from build123d import *

# Parameters (mm, degrees)
SKETCH1_W           = 58
SKETCH1_H           = 90
SKETCH1_W_2         = 46
SKETCH1_H_2         = 78
BOSS_EXTRUDE1_DEPTH = 3
BOSS_EXTRUDE2_DEPTH = 6
SKETCH3_R           = 2.05
CUT_EXTRUDE1_DEPTH  = 108.447661678
SKETCH4_R           = 2.05
CUT_EXTRUDE2_DEPTH  = 108.447661678
FILLET1_R           = 2
FILLET2_R           = 2
SKETCH5_W           = 8
SKETCH5_H           = 3
BOSS_EXTRUDE3_DEPTH = 3
SKETCH6_R           = 2.05
CUT_EXTRUDE3_DEPTH  = 3
FILLET3_R           = 3
SKETCH7_W           = 3
SKETCH7_H           = 8
BOSS_EXTRUDE4_DEPTH = 3
SKETCH8_R           = 2.05
CUT_EXTRUDE4_DEPTH  = 108.238052948
FILLET4_R           = 3


with BuildPart() as part:
    # Sketch1 → Boss-Extrude1 (new body)
    with BuildSketch(Plane(origin=(0, 0, 0), x_dir=(1, 0, 0), z_dir=(0, 1, 0))):
        with Locations((29, -45)):
            Rectangle(SKETCH1_W, SKETCH1_H)
        with Locations((29, -45)):
            Rectangle(SKETCH1_W_2, SKETCH1_H_2, mode=Mode.SUBTRACT)
    extrude(amount=BOSS_EXTRUDE1_DEPTH)

    # Sketch2 → Boss-Extrude2 (add)
    with BuildSketch(Plane(origin=(0, 3, 0), x_dir=(1, 0, 0), z_dir=(0, 1, 0))):
        Polygon((46, -84), (46, -90), (58, -90), (58, -78), (52, -78), (52, -84), align=None)
        Polygon((52, -12), (58, -12), (58, 0), (46, 0), (46, -6), (52, -6), align=None)
        Polygon((0, 0), (0, -12), (6, -12), (6, -6), (12, -6), (12, 0), align=None)
        Polygon((0, -90), (12, -90), (12, -84), (6, -84), (6, -78), (0, -78), align=None)
    extrude(amount=BOSS_EXTRUDE2_DEPTH)

    # Sketch3 → Cut-Extrude1 (cut, through all)
    with BuildSketch(Plane.ZY):
        with Locations((9, 6)):
            Circle(SKETCH3_R)
        with Locations((81, 6)):
            Circle(SKETCH3_R)
    extrude(amount=-CUT_EXTRUDE1_DEPTH, mode=Mode.SUBTRACT)

    # Sketch4 → Cut-Extrude2 (cut, through all)
    with BuildSketch(Plane(origin=(0, 0, 0), x_dir=(-1, 0, 0), z_dir=(0, 0, -1))):
        with Locations((-49, 6)):
            Circle(SKETCH4_R)
        with Locations((-9, 6)):
            Circle(SKETCH4_R)
    extrude(amount=-CUT_EXTRUDE2_DEPTH, mode=Mode.SUBTRACT)

    # Fillet1
    fillet1_edges = [part.edges().sort_by_distance(p)[0] for p in [
        (55, 9, 78),
        (55, 9, 12),
        (46, 9, 3),
        (3, 9, 12),
        (12, 9, 3),
        (3, 9, 78),
        (12, 9, 87),
    ]]
    fillet(fillet1_edges, radius=FILLET1_R)

    # Fillet2
    fillet2_edges = [part.edges().sort_by_distance(p)[0] for p in [
        (0, 4.5, 0),
        (58, 4.5, 0),
        (58, 4.5, 90),
        (0, 4.5, 90),
    ]]
    fillet(fillet2_edges, radius=FILLET2_R)

    # Sketch5 → Boss-Extrude3 (add)
    with BuildSketch(Plane.XZ):
        with Locations((29, 7.5)):
            Rectangle(SKETCH5_W, SKETCH5_H)
        with Locations((29, 82.5)):
            Rectangle(SKETCH5_W, SKETCH5_H)
    extrude(amount=-BOSS_EXTRUDE3_DEPTH)

    # Sketch6 → Cut-Extrude3 (cut)
    with BuildSketch(Plane.XZ):
        with Locations(Location((29, 85.5, 0), (0, 0, 270))):
            Circle(SKETCH6_R)
        with Locations(Location((29, 4.5, 0), (0, 0, 270))):
            Circle(SKETCH6_R)
    extrude(amount=-CUT_EXTRUDE3_DEPTH, mode=Mode.SUBTRACT)

    # Fillet3
    fillet3_edges = [part.edges().sort_by_distance(p)[0] for p in [
        (33, 1.5, 81),
        (25, 1.5, 81),
        (33, 1.5, 9),
        (25, 1.5, 9),
    ]]
    fillet(fillet3_edges, radius=FILLET3_R - 0.0001)  # a hair under: the kernel refuses the full size

    # Sketch7 → Boss-Extrude4 (add)
    with BuildSketch(Plane.XZ):
        with Locations((50.5, 45)):
            Rectangle(SKETCH7_W, SKETCH7_H)
        with Locations((7.5, 45)):
            Rectangle(SKETCH7_W, SKETCH7_H)
    extrude(amount=-BOSS_EXTRUDE4_DEPTH)

    # Sketch8 → Cut-Extrude4 (cut, through all)
    with BuildSketch(Plane(origin=(0, 3, 0), x_dir=(1, 0, 0), z_dir=(0, 1, 0))):
        with Locations(Location((4.5, -45, 0), (0, 0, 270))):
            Circle(SKETCH8_R)
        with Locations(Location((53.5, -45, 0), (0, 0, 270))):
            Circle(SKETCH8_R)
    extrude(amount=-CUT_EXTRUDE4_DEPTH, mode=Mode.SUBTRACT)

    # Fillet4
    fillet4_edges = [part.edges().sort_by_distance(p)[0] for p in [
        (49, 1.5, 41),
        (49, 1.5, 49),
        (9, 1.5, 41),
        (9, 1.5, 49),
    ]]
    fillet(fillet4_edges, radius=FILLET4_R - 0.0001)  # a hair under: the kernel refuses the full size


solid = part.part
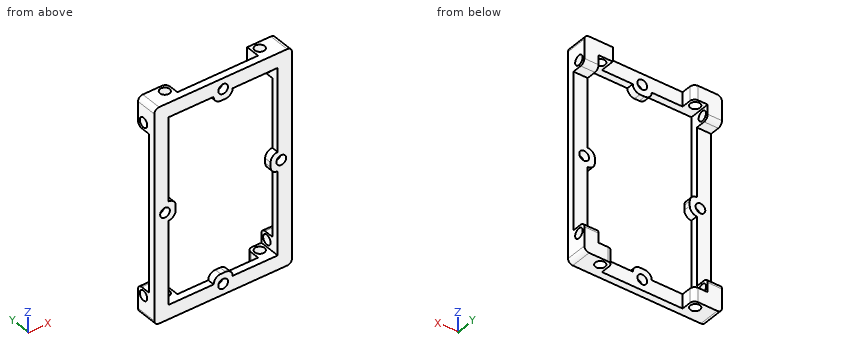
The listing builds one solid part. Answer for the finished solid, in the listing's coordinates (mm). Coordinates: 2 decimals unless noted, no trailing zeros. Write each loop counter-clockwise with the first axis right and the second up, starting at its lowest first coordinate (ties: lowest second). Pieces come first, ordered by that corner, then holes. Notation, with made-up numbers: M -10,83.25 L -2,83.25 A31 ccw -2,108.25 Z; hole C 87,35.25 d7. An arc over 180 degrees is marked long. Write each question's results on one line, items separated by ' | '.
Item 1: Consider probe 1 along X at (y, z) = (0.85, 45); probe 2 along X at (y, z) = (2.5, 14); probe 3 along Z at (x, y) = (50.5, 7.75). Determine where each line is inside the solid, lowest interval first. Write a range as [from, to].
Answer below:
probe 1: [0, 2.45], [6.55, 9], [49, 51.45], [55.55, 58] | probe 2: [0, 6], [52, 58] | probe 3: [0, 6], [84, 90]
Item 2: The part is cut by section A-A on z = 4.5. Determine the outline of the cut face in (x, y), and give its area (3 significant figures).
Answer below:
outline: M 0,0 L 26.95,0 L 26.95,3 L 12,3 L 12,7 A2 ccw 10,9 L 0,9 Z; M 31.05,0 L 58,0 L 58,9 L 48,9 A2 ccw 46,7 L 46,3 L 31.05,3 Z; hole C 9,6 d4.1; hole C 49,6 d4.1 | area: 278 mm2
Item 3: Given P1, Ø6, axis at x = 35.5, z = 78.5, coming from the -Y side; P2, Ø2.5, axis at x = 4, z = 54, coming from the +Y side; P3, Ø4.5, axis at x = 16, y = 3.5, coming from the -Z side, each flat-ended and moving along its own axis, determine where each tip first touches the part or whether it passes through.
Answer below:
P1: through | P2: y = 3 | P3: z = 0
Item 4: The part is cut by section B-B on x = 40.5. Determine the outline of the cut face in (y, z), and give its area (3 significant figures).
Answer below:
outline: M 0,0 L 3,0 L 3,6 L 0,6 Z; M 0,84 L 3,84 L 3,90 L 0,90 Z | area: 36.0 mm2
Item 5: The part is cut by section C-C on z = 25.5. Determine the outline of the cut face in (x, y).
Answer below:
outline: M 0,0 L 6,0 L 6,3 L 0,3 Z; M 52,0 L 58,0 L 58,3 L 52,3 Z
Item 6: The part is cut by section D-D on x = 4.5. Determine the outline of the cut face in (y, z), and give its area (3 significant figures).
Answer below:
outline: M 0,0 L 9,0 L 9,10 A2 ccw 7,12 L 3,12 L 3,42.95 L 0,42.95 Z; M 0,47.05 L 3,47.05 L 3,78 L 7,78 A2 ccw 9,80 L 9,90 L 0,90 Z; hole C 6,9 d4.1; hole C 6,81 d4.1 | area: 374 mm2
